Autodesk Inventor part; units mm, degrees
ref_plane "Start Plane" through (0, 0, 25.13) normal (0, 0, 1) x (1, 0, 0)
ref_plane "End Plane" through (0, 0, 1974.87) normal (0, 0, 1) x (1, 0, 0)
ref_plane "Work Plane4" through (0, 200, 25.13) normal (0, 0, -1) x (-1, 0, 0)
ref_plane "Start Plane" through (0, 0, 25.13) normal (0, 0, 1) x (1, 0, 0)
ref_plane "End Plane" through (0, 0, 1974.87) normal (0, 0, 1) x (1, 0, 0)
sketch "Sketch" plane through (0, 0, 0) normal (0, 0, 1) x (1, 0, 0)
  circle A0 centre (0, 0) radius 20.447
  circle A1 centre (0, 0) radius 24.13
  dimension "d0" = 48.26
  dimension "d1" = 3.683
extrude "Body" add sketch "Sketch" along normal up to surface (1949.74 mm away) from surface at 25.13
sketch "Sketch3" plane through (0, 0, 0) normal (0, 0, 1) x (1, 0, 0)
  line L0 (0, 0) -> (10, 0)
ref_plane "Work Plane3" through (0, 0, 0) normal (0, -1, 0) x (1, 0, 0)
ref_plane "Work Plane4" through (0, 200, 25.13) normal (0, 0, -1) x (-1, 0, 0)
split "Split1" plane through (0, 200, 25.13) removes the side toward (0, 0, -1)
ref_plane "Work Plane5" through (0, 200, 1974.87) normal (0, 0, 1) x (1, 0, 0)
split "Split2" plane through (0, 200, 1974.87) removes the side toward (0, 0, 1)
sketch "Sketch4" plane through (0, 0, 0) normal (0, -1, 0) x (1, 0, 0)
  line L0 (-2, 25.13) -> (12, 25.13)
  line L1 (-2, 1974.87) -> (12, 1974.87)
  dimension "d7" = 1949.74
equation "\"d0\" = G_H"
equation "\"d1\" = G_T"
equation "\"d2\" = G_L"
equation "\"G_H\" = 48.26"
equation "\"G_T\" = 3.683"
equation "\"G_L\" = d7"
equation "\"G_OFFSET_START\" = -25.13"
equation "\"G_OFFSET_END\" = -25.13"
equation "\"d4\" = -G_OFFSET_START"
equation "\"d5\" = G_OFFSET_END + B_L"
properties part number "ANSI - 1 1/2 x 0.145 - 76.761" material "Steel, Mild"
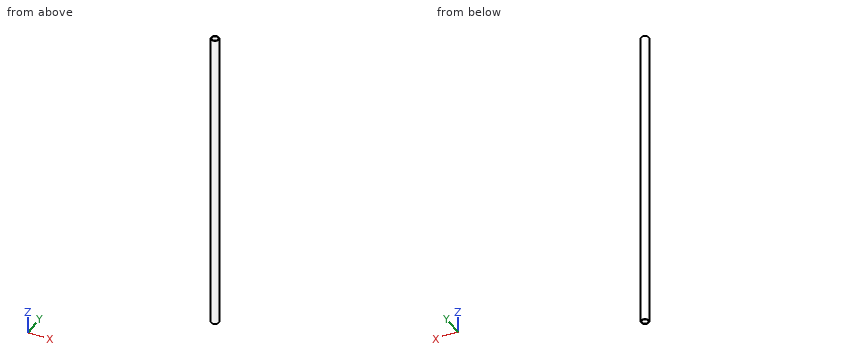
CAD build for the part. Positions are in the model's coordinates, mm. Round coordinates to 2 decimals unless told otherwise and drop trailing zeros. Order: outer loops, then holes, each group sorted by start corner. A loop starts at its lowest first (then second) coordinate and runs counter-clockwise, first axis right, second up.
Item 1: Probe line 1 along Y through (x, z) = (0, 1511); line 2 along X through (y, z) = (-0.5, 167); line 3 along X through (y, z) = (-17, 1105.5). List the from-to ranges inside material, lowest first.
Item 2: Pin check, flat tips, straight feed: pin 1 (12 mm diameter, centred on x = -4.5, z = 1110.5, fed in from -Y); pin 2 (6 mm diameter, centred on x = -8.5, z = 377.5, fed in from -Y); pin 3 (2 mm diameter, centred on x = 18.5, z = 734.5, fed in from -Y). Stop position of each tip, or through.
Item 3: Saw through at A-A on y = 0. Write the cut outline in (x, z), then the cut area to 3 significant figures.
Item 4: Saw through at C-C on z = 1491.5. Write the cut outline in (x, y), then the cut area to 3 significant figures.
Reported:
1. line 1: y = -24.13 to -20.45, 20.45 to 24.13
1. line 2: x = -24.12 to -20.44, 20.44 to 24.12
1. line 3: x = -17.12 to -11.36, 11.36 to 17.12
2. pin 1: stops at y = -24.13
2. pin 2: stops at y = -23.49
2. pin 3: stops at y = -16.61
3. outline: (-24.13, 25.13) - (-20.45, 25.13) - (-20.45, 1974.87) - (-24.13, 1974.87) - close; (20.45, 25.13) - (24.13, 25.13) - (24.13, 1974.87) - (20.45, 1974.87) - close
3. area: 14,400 mm2
4. outline: circle Ø48.26 at (0, 0); hole circle Ø40.89 at (0, 0)
4. area: 516 mm2
